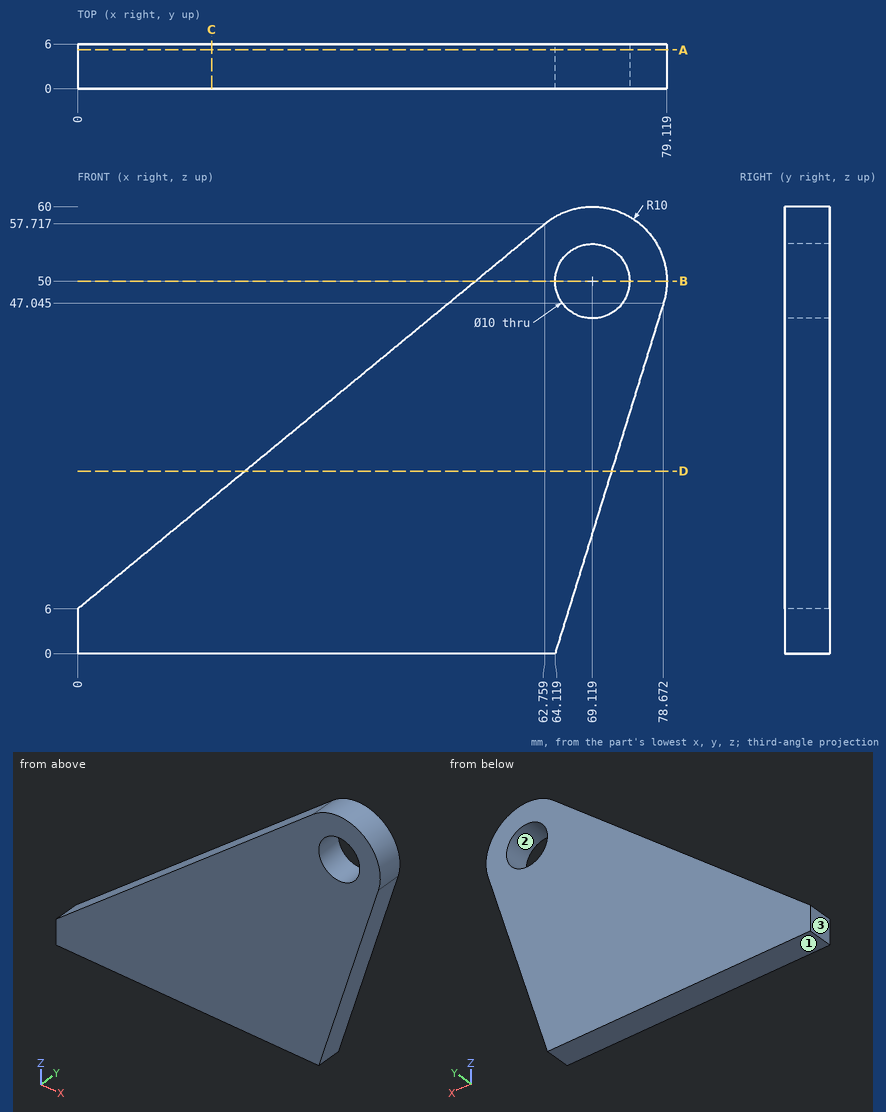
Can you work these out from the drawing? Everything is in mm from the part's minimum corner. Give positions to 0.01 mm unless a question says otherwise; leave off trailing zeros. Loops run counter-clockwise (first coordinate to the right, second up) from the corner with the lowest first, then second, coordinate; pieces in that order, holes last. Notation, with made-up numbers: M 74,25 L 90,25 A12 cw 90,41 Z; hole C -3.75,26 d10. An arc over 180 degrees is marked long. Use CSV: the item, a comma, the result in double quotes. Start each with the question number.
1. If we mould it in two halves opening along X, with no side actions, what happens to the marked faces 1, 2 and 3? For each: released by +X, released by -X, zero draft, split by the parting line, or undercut.
2. Imagine slicing it at A-A, the plane y = 5.2. Write out the boundary of the cut face in (x, z) (1 decimal), plus the area to 3 significant figures.
3. Imagine slicing it at C-C, the plane x = 18. Write out the boundary of the cut face in (y, z).
4. Imagine slicing it at D-D, the plane z = 24.5. Write out the boundary of the cut face in (x, y).
5. If I drill on L1, parallel to X at y = 5.25, z = 45.5 (1 decimal); L2, parallel to X at y = 3, z = 27.5 (1 decimal); L3, parallel to X at y = 5.7, z = 12, over which ranges is the centre line in solid material (lowest first)?
6. For P1, Ø2, axis at y = 4, z = 42.5, coming from the -X side, with a flat end and sliding along its axis, tell me the tip position at first contact or that it passes through.
7. Imagine slicing it at B-B, the plane z = 50. Write out the boundary of the cut face in (x, y).
Response values:
1,face 1,"zero draft"
1,face 2,"undercut"
1,face 3,"released by -X"
2,outline,"M 0,0 L 64.1,0 L 78.7,47 A10 ccw 62.8,57.7 L 0,6 Z; hole C 69.1,50 d10"
2,area,"2,510 mm^2"
3,outline,"M 0,0 L 6,0 L 6,20.83 L 0,20.83 Z"
4,outline,"M 22.45,0 L 71.7,0 L 71.7,6 L 22.45,6 Z"
5,L1,"47.9 to 66.9, 71.3 to 78.2"
5,L2,"26.1 to 72.6"
5,L3,"7.28 to 67.83"
6,P1,"x = 43.08"
7,outline,"M 53.39,0 L 64.12,0 L 64.12,6 L 53.39,6 Z; M 74.12,0 L 79.12,0 L 79.12,6 L 74.12,6 Z"
